Autodesk Inventor part; units mm, degrees
ref_plane "YZ Plane" through (0, 0, 0) normal (1, 0, 0) x (0, 1, 0)
ref_plane "XZ Plane" through (0, 0, 0) normal (0, 1, 0) x (-1, 0, 0)
ref_plane "XY Plane" through (0, 0, 0) normal (0, 0, 1) x (1, 0, 0)
sketch "Sketch1" plane through (0, 0, 0) normal (0, 1, 0) x (-1, 0, 0)
  circle A0 centre (0, 0) radius 7.9375
  line L0 (0, -7.9375) -> (0, -17.7165)
  line L1 (0, -17.7165) -> (0, -33.5915)
  circle A1 centre (0, -25.654) radius 7.9375
  line L2 (0, 0) -> (0, -25.654) construction
  line L3 (-7.9375, 0) -> (-7.9375, -25.654)
  line L4 (7.9375, -25.654) -> (7.9375, 0)
  arc A2 (7.9375, 0) -> (-7.9375, 0) centre (0, 0) ccw
  arc A3 (-7.9375, -25.654) -> (7.9375, -25.654) centre (0, -25.654) ccw
  line L5 (10.4775, 0) -> (10.4775, -25.654)
  arc A4 (-10.4775, -25.654) -> (10.4775, -25.654) centre (0, -25.654) ccw
  line L6 (-10.4775, -25.654) -> (-10.4775, 0)
  arc A5 (10.4775, 0) -> (-10.4775, 0) centre (0, 0) ccw
  point P0 (0, -12.827)
  dimension "d0" = 15.875
  dimension "d1" = 9.779
  dimension "d2" = 15.875
  dimension "d3" = 2.54
extrude "Extrusion1" add sketch "Sketch1" along normal blind 1.27 contours L4 A1 L0 A0 | A0 L0 A1 L3 | L5 A4 L6 A5
sketch "Sketch2" plane through (10.4775, 0, 0) normal (1, 0, 0) x (0, 0, -1)
  line L0 (25.654, 0) -> (0, 0)
  line L1 (12.827, 0) -> (12.827, -2.54)
  line L2 (12.827, -2.54) -> (10.287, 0)
  line L3 (12.827, -2.54) -> (15.367, 0)
  dimension "d6" = 2.54
  dimension "d7" = 45
extrude "Extrusion2" add sketch "Sketch2" against normal up to surface (20.955 mm away)
fillet "Fillet1" radius 0.762 3 edges at (0, 0, -15.367) (0, -2.54, -12.827) (0, 0, -10.287)
chamfer "Chamfer1" distance 1.27 angle 45 4 edges at (10.4775, 1.27, -12.827) (0, 1.27, -36.1315) (-10.4775, 1.27, -12.827) (0, 1.27, 10.4775)
properties part number "Ultrasonic Sensor Cover_3DPrint"
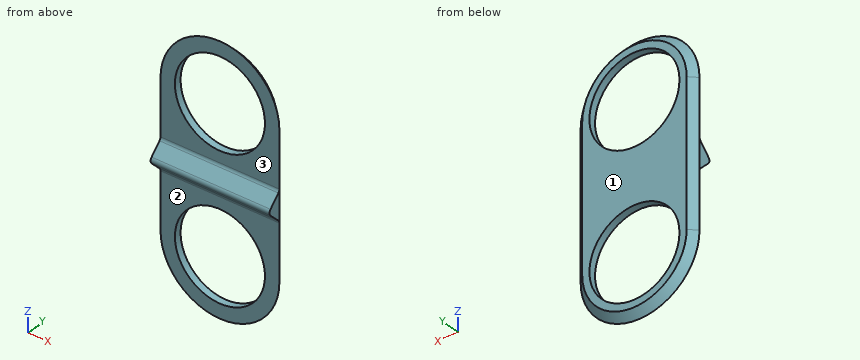
CAD build for the part. Positions are in the model's coordinates, mm. Face numbers are marked on the shaded views. A direction names the side the tool comes from. Round coordinates to 2 decimals unless told otherwise and drop trailing zeros. Write each loop counter-clockwise with the first axis right and the second up, starting at its lowest first coordinate (ties: lowest second). Pieces come first, ordered by that corner, then holes. Notation, with made-up numbers: M 75.25,-33.5 L 110.25,-33.5 A18 cw 110.25,-18.5 Z; hole C 47,17.25 d9. An arc over 180 degrees is marked long. Use a Markdown table: item, result. Add a question column.
1. Flat gauge pin, fed straight in: P1, Ø2, axis at x = -5, z = -8.5, coming from the -Y side. Where does the tip first touch, or does it go through?
2. Slice it at B-B on y = 0.55. Give the cut face in (x, z) (1 decimal).
3. 3-axis set-ups, long thin cutter, end or side, ignore diameter. For the marked faces 1, 2 and 3: which of +Z, -Z, +X, -X, +Y, -Y reach the whole face in a straight line?
4. Drill centre lines: probe 1 along Z at (x, y) = (0, 0.85); probe 2 along Z at (x, y) = (0.75, 0.8); probe 3 along Y at (x, z) = (-5.25, -33). Where is each one in solid material? Low to high.
5. Slice it at A-A on x = 0. Give the number of separate pieces and of enclosed holes in the cut face, then the cut area to 3 significant figures.
Reply:
| question | item | result |
|---|---|---|
| 1 | P1 | stops at y = 0 |
| 2 | outline | M -9.9,-25.7 A9.9 ccw 9.9,-25.7 L 9.9,0 A9.9 ccw -9.9,0 Z; hole C 0,-25.7 d15.9; hole C 0,0 d15.9 |
| 3 | face 1 | +Z, -Z, +X, -X, +Y |
| 3 | face 2 | -Z, +X, -X, -Y |
| 3 | face 3 | +Z, +X, -X, -Y |
| 4 | probe 1 | z = -35.28 to -33.59, -17.72 to -7.94, 7.94 to 9.63 |
| 4 | probe 2 | z = -35.3 to -33.56, -17.75 to -7.9, 7.9 to 9.65 |
| 4 | probe 3 | y = 0 to 1.27 |
| 5 | separate pieces | 3 |
| 5 | enclosed holes | 0 |
| 5 | area | 23.6 mm^2 |
